The figure shows three views and two pictorial views of one solid part (mm, origin at its lowest corner). Answer the questions. Give positions to 0.01 mm unless a question says otherwise; leave off trailing zeros. Order: outer loops, then holes, each group sorted by start corner. A loop starts at its lowest first (then second) coordinate and runs counter-clockwise, first axis right, second up. Notation, with made-up numbers: M 43,38.25 L 50,38.25 A26 cw 50,56.25 Z; hole C -36,66.5 d4. An arc over 180 degrees is marked long. One line per item, written item: value.
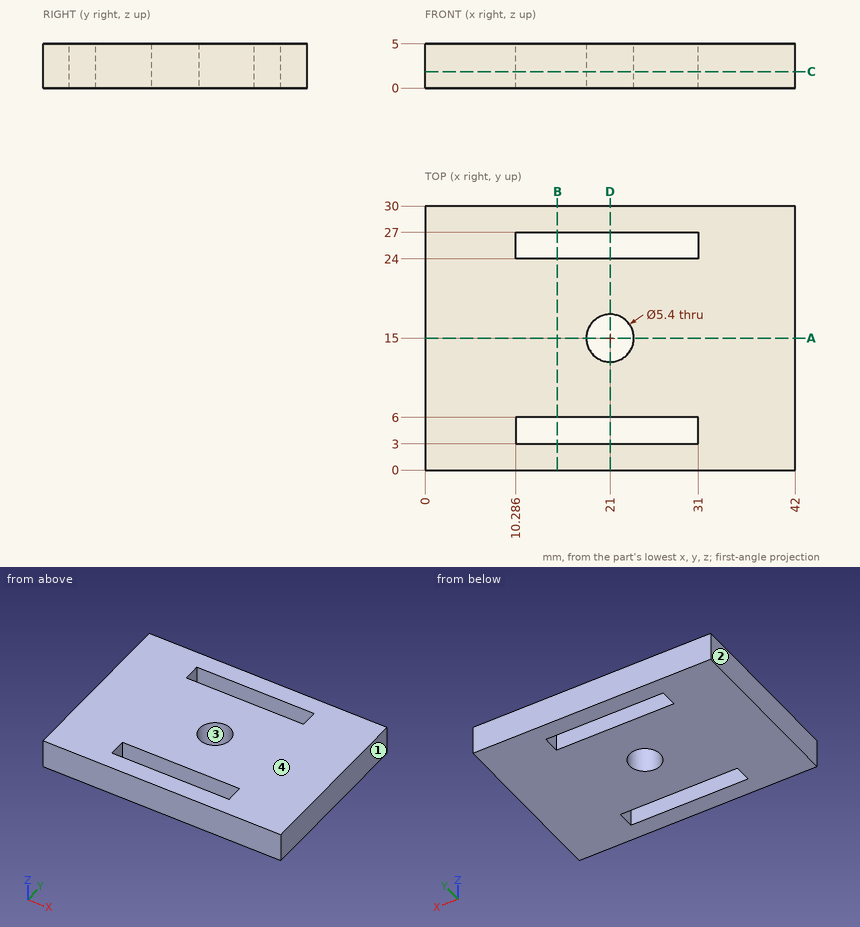
1) Determine the mould class of the marked faces 1, 2, 3 and 4 for opening direction X: +X half, -X half, draft (parallel to the pull), parting line (faces both ways), or undercut.
Reported:
face 1: +X half
face 2: -X half
face 3: undercut
face 4: draft
2) Find section B-B, the plane x = 15. Write down the section's boundary in (y, z).
Reported:
outline: M 0,0 L 3,0 L 3,5 L 0,5 Z; M 6,0 L 24,0 L 24,5 L 6,5 Z; M 27,0 L 30,0 L 30,5 L 27,5 Z
3) Consider probe 1 along Y at (x, z) = (15, 0.35); probe 2 along Y at (x, z) = (21, 1.75); probe 3 along X at (y, z) = (5.75, 4.6). Determine where each line is inside the solid, lowest interval first.
Reported:
probe 1: y = 0 to 3, 6 to 24, 27 to 30
probe 2: y = 0 to 3, 6 to 12.3, 17.7 to 24, 27 to 30
probe 3: x = 0 to 10.29, 31 to 42
4) Find section D-D, the plane x = 21. Write down the section's boundary in (y, z).
Reported:
outline: M 0,0 L 3,0 L 3,5 L 0,5 Z; M 6,0 L 12.3,0 L 12.3,5 L 6,5 Z; M 17.7,0 L 24,0 L 24,5 L 17.7,5 Z; M 27,0 L 30,0 L 30,5 L 27,5 Z
5) Find section C-C, the plane z = 1.85. Write down the section's boundary in (x, y), plus the area to 3 significant figures.
Reported:
outline: M 0,0 L 42,0 L 42,30 L 0,30 Z; hole M 10.29,3 L 31,3 L 31,6 L 10.29,6 Z; hole M 10.29,24 L 31,24 L 31,27 L 10.29,27 Z; hole C 21,15 d5.4
area: 1,110 mm^2
6) Find section A-A, the plane y = 15. Write down the section's boundary in (x, z).
Reported:
outline: M 0,0 L 18.3,0 L 18.3,5 L 0,5 Z; M 23.7,0 L 42,0 L 42,5 L 23.7,5 Z
7) This flat-tipped pin is pushed along its axis until it touches: pin 1 Ø1.5 at (x, z) = (20, 2) entering from -Y. Where does it stop, or does it pass through?
Reported:
pin 1: stops at y = 0
